Print and shaded views of the part. All mm, measured from the part's lowest x, y and z. A direction names the side the tool comes from. Round coordinates to 2 decimals unless told otherwise and drop trailing zeros. Order: outer loops, then holes, each group sorted by start corner. A loop starts at its lowest first (then second) coordinate and runs counter-clockwise, first axis right, second up. Notation, with made-up numbers: M -37,36.5 L 12,36.5 A27 cw 12,57.5 Z; hole C 30.5,39 d6. An arc over 180 degrees is marked long. Write each question's results on one line, items separated by ' | '. Start each with the question number.
1. Band-saw the part on D-D, the plane z = 21.5. List the corners of the cut face in (x, y), then the cut area to 3 significant figures.
2. Which spindle directions (+Z, -Z, +X, -X, +Y, -Y) get a long thin tool onto all of the face, cutting with end or side? Do the marked faces 1, 2 and 3. Say none if no direction does.
3. Probe L1, parallel to X at y = 5.5, z = 16.5; L2, parallel to Z at x = 30, y = 4.5; L3, parallel to Z at x = 6.5, y = 6.25 (1 decimal). List the from-to ranges inside material, lowest first. Write a range as [from, to].
4. Two-plate mould, pull along X, no slides. Class the marked faces 4, 5 and 6: +X half, -X half, draft (parallel to the pull), parting line (faces both ways), or undercut.
5. Band-saw the part on A-A, the plane z = 7. Give the number of separate pieces and of enclosed holes in the cut face, then the cut area to 3 significant figures.
6. Drop flat-ended pins along their axis: pin 1 Ø6.5 at (y, z) = (14.5, 17) entering from +X; pin 2 Ø3 at (y, z) = (15.45, 18) entering from +X; pin 3 Ø6.5 at (y, z) = (15.45, 7) entering from +X; pin 4 Ø6 at (x, z) = (4.5, 14.5) entering from +Y. Give the stop position or say it passes through.
7. Band-saw the part on B-B, the plane x = 20.5. List the corners of the cut face in (y, z), then the cut area to 3 significant figures.
8. Band-saw the part on C-C, the plane y = 2.25. List the corners of the cut face in (x, z) (1 decimal), then the cut area to 3 significant figures.
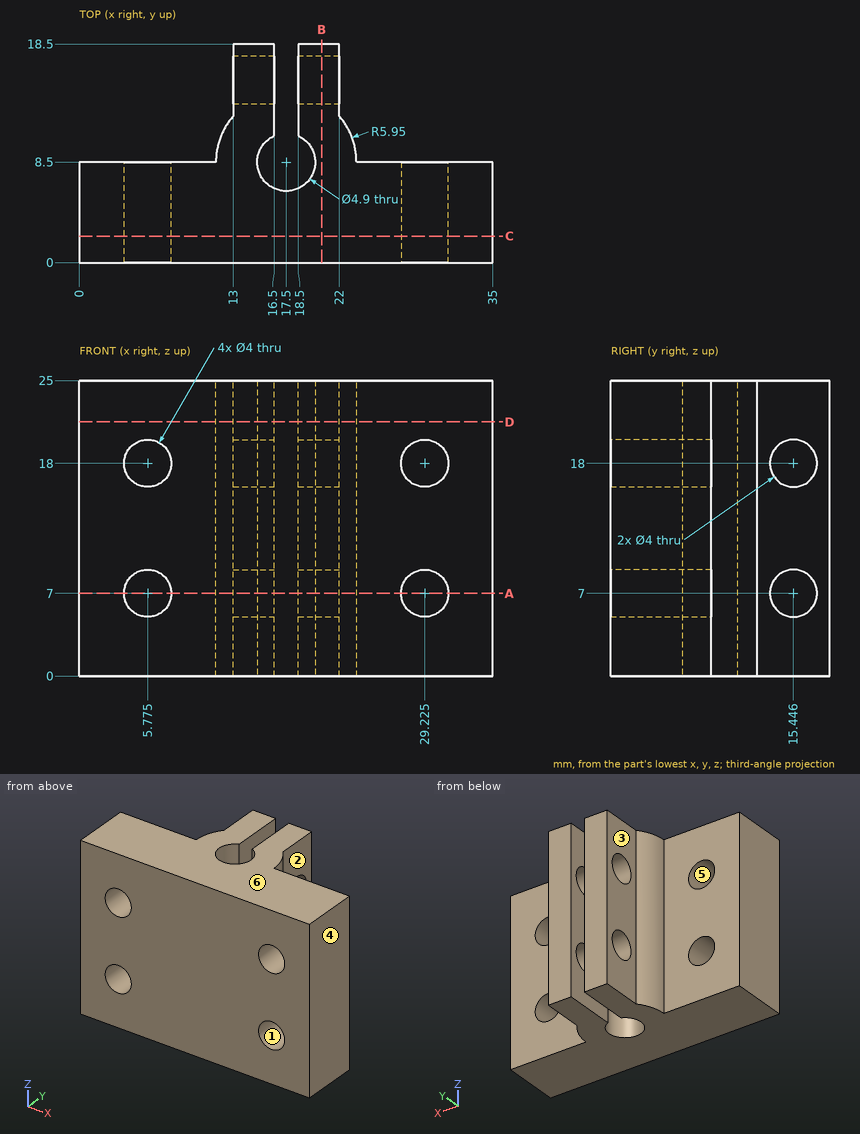
Solution:
1) outline: M 0,0 L 35,0 L 35,8.5 L 23.45,8.5 A5.95 ccw 22,12.39 L 22,18.5 L 18.5,18.5 L 18.5,10.74 A2.45 cw long 16.5,10.74 L 16.5,18.5 L 13,18.5 L 13,12.39 A5.95 ccw 11.55,8.5 L 0,8.5 Z | area: 361 mm^2
2) face 1: +Y, -Y | face 2: +Z, -Z, +X, +Y | face 3: +Z, -Z, -X, +Y
3) L1: [0, 4.45], [7.1, 27.9], [30.55, 35] | L2: [0, 5.16], [8.84, 16.16], [19.84, 25] | L3: [0, 5.1], [8.9, 16.1], [19.9, 25]
4) face 4: +X half | face 5: undercut | face 6: draft
5) separate pieces: 5 | enclosed holes: 0 | area: 265 mm^2
6) pin 1: x = 22.78 | pin 2: through | pin 3: x = 22.16 | pin 4: y = 8.5
7) outline: M 0,0 L 18.5,0 L 18.5,25 L 0,25 Z; hole C 15.45,7 d4; hole C 15.45,18 d4 | area: 437 mm^2
8) outline: M 0,0 L 35,0 L 35,25 L 0,25 Z; hole C 5.8,7 d4; hole C 5.8,18 d4; hole C 29.2,7 d4; hole C 29.2,18 d4 | area: 825 mm^2
